```python
from build123d import *

# Parameters (mm, degrees)
F0_R        = 16.3870034363
F1_DEPTH    = 25.4
F2_T1_DEPTH = 116.4008158105
F2_T3_DEPTH = 104.7146316577
F2_T5_DEPTH = 112.6871608157
F2_T7_DEPTH = 79.0886539925
F3_T1_DEPTH = 116.4008158105
F3_T3_DEPTH = 104.7146316577
F3_T5_DEPTH = 112.6871608157
F3_T7_DEPTH = 79.0886539925


# Not quite as in the source:
# - a fillet or chamfer that OpenCascade refuses, or shapes differently, is made with other operations: its cross-section is extruded or revolved along the edge and cut away or added


with BuildPart() as f1:
    # F0 (on Top) → F1 (new body)
    with BuildSketch(Plane.XY):
        Polygon((27.1920096129, 8.1148929894), (-59.3668520451, 33.7408706546), (-59.3668520451, -44.8454618454), (27.1920096129, -44.8454618454), align=None)
        with Locations((0, -4.4133625925)):
            Circle(F0_R, mode=Mode.SUBTRACT)
    extrude(amount=F1_DEPTH)

    # F2: chamfer of 5.08 on 5 edges, made by hand

    # F2_s2 → F2_t1 (cut)
    with BuildSketch(Plane(origin=(35.3186398876, -10.4561758275, 0), x_dir=(0, 0, 1), z_dir=(-0.9588617319, 0.2838735267, 0))):
        Polygon((20.32, 15.5001520123), (25.4, 10.4201520123), (25.4, 15.5001520123), align=None)
    extrude(amount=F2_T1_DEPTH, mode=Mode.SUBTRACT)

    # F2_s4 → F2_t3 (cut)
    with BuildSketch(Plane.XZ.offset(-46.8050202334)):
        Polygon((-59.3668520451, 20.32), (-54.2868520451, 25.4), (-59.3668520451, 25.4), align=None)
    extrude(amount=F2_T3_DEPTH, mode=Mode.SUBTRACT)

    # F2_s6 → F2_t5 (cut)
    with BuildSketch(Plane.YZ.offset(-72.4310016239)):
        Polygon((-44.8454618454, 20.32), (-39.7654618454, 25.4), (-44.8454618454, 25.4), align=None)
    extrude(amount=F2_T5_DEPTH, mode=Mode.SUBTRACT)

    # F2_s8 → F2_t7 (cut)
    with BuildSketch(Plane.XZ.offset(-21.1790425683)):
        Polygon((27.1920096129, 20.32), (22.1120096129, 25.4), (27.1920096129, 25.4), align=None)
    extrude(amount=F2_T7_DEPTH, mode=Mode.SUBTRACT)

    # F2_s9 → F2_t10 (revolve, cut)
    with BuildSketch(Plane.XZ.offset(4.4133625925)):
        Polygon((16.3870034363, 20.32), (21.4670034363, 25.4), (16.3870034363, 25.4), align=None)
    revolve(axis=Axis((0, -4.4133625925, 25.4), (0, 0, 1)), mode=Mode.SUBTRACT)

    # F3: chamfer of 5.08 on 5 edges, made by hand

    # F3_s2 → F3_t1 (cut)
    with BuildSketch(Plane(origin=(35.3186398876, -10.4561758275, 0), x_dir=(0, 0, 1), z_dir=(-0.9588617319, 0.2838735267, 0))):
        Polygon((5.08, 15.5001520123), (0, 10.4201520123), (0, 15.5001520123), align=None)
    extrude(amount=F3_T1_DEPTH, mode=Mode.SUBTRACT)

    # F3_s4 → F3_t3 (cut)
    with BuildSketch(Plane.XZ.offset(-46.8050202334)):
        Polygon((-54.2868520451, 0), (-59.3668520451, 5.08), (-59.3668520451, 0), align=None)
    extrude(amount=F3_T3_DEPTH, mode=Mode.SUBTRACT)

    # F3_s6 → F3_t5 (cut)
    with BuildSketch(Plane.YZ.offset(-72.4310016239)):
        Polygon((-39.7654618454, 0), (-44.8454618454, 5.08), (-44.8454618454, 0), align=None)
    extrude(amount=F3_T5_DEPTH, mode=Mode.SUBTRACT)

    # F3_s8 → F3_t7 (cut)
    with BuildSketch(Plane.XZ.offset(-21.1790425683)):
        Polygon((22.1120096129, 0), (27.1920096129, 5.08), (27.1920096129, 0), align=None)
    extrude(amount=F3_T7_DEPTH, mode=Mode.SUBTRACT)

    # F3_s9 → F3_t10 (revolve, cut)
    with BuildSketch(Plane.XZ.offset(4.4133625925)):
        Polygon((21.4670034363, 0), (16.3870034363, 5.08), (16.3870034363, 0), align=None)
    revolve(axis=Axis((0, -4.4133625925, 0), (0, 0, 1)), mode=Mode.SUBTRACT)


solid = f1.part
```
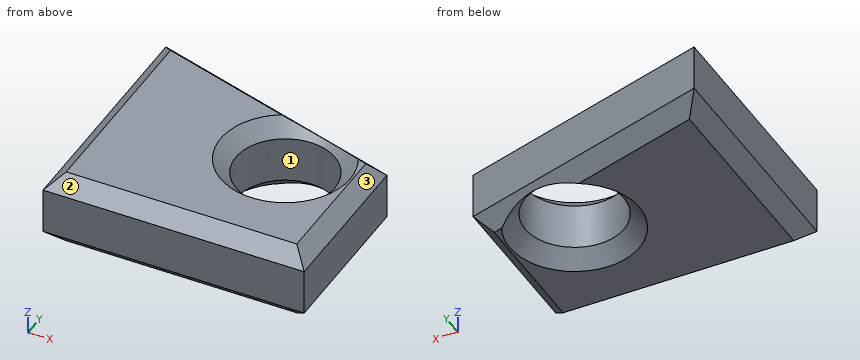
Part model, mm, in its own coordinate system. Face numbers are marked on the shaded views. Round coordinates to 2 decimals unless told otherwise and drop trailing zeros. Loops run counter-clockwise (first coordinate to the right, second up) from the corner with the lowest first, then second, coordinate; pieces in that order, holes last.
Item 1: Cut at C-C, the plane x = -49.5. Give the cut face in (y, z).
Item 2: Drop flat-ended pins along their axis: P1, Ø3, axis at x = 8, y = -18, coming from the +Z side; P2, Ø2, axis at x = -11.5, z = 10.5, coming from the +Y side; P3, Ø5, axis at x = -2.5, z = 7.5, coming from the +Y side. Give the stop position or say it passes through.
Item 3: Cut at B-B, the plane y = -33. Give the cut face in (x, z), then the cut area to 3 significant figures.
Item 4: Drill centre lines: line 1 (Y direction, x = 0, z = 8.75); line 2 (X direction, y = -3, z = 8.25); line 3 (X direction, y = 8, z = 16.5). Where is each one in solid material? Low to high.
Item 5: Cut at D-D, the plane z = 8.5. Give the cut face in (x, y), then the cut area to 3 significant figures.
Item 6: Mould opens along Y. For the marked faces 1, 2 and 3 say: +Y half, -Y half, draft (parallel to the pull), parting line (faces both ways), or undercut.
Item 7: Cut at A-A, the plane x = 0. Give the cut face in (y, z), then the cut area to 3 significant figures.
A:
1. outline: (-44.85, 5.08) - (-39.77, 0) - (25.52, 0) - (30.82, 5.08) - (30.82, 20.32) - (25.52, 25.4) - (-39.77, 25.4) - (-44.85, 20.32) - close
2. P1: stops at z = 21.2
2. P2: stops at y = 19.87
2. P3: stops at y = 17.65
3. outline: (-59.37, 5.08) - (-54.29, 0) - (22.11, 0) - (27.19, 5.08) - (27.19, 20.32) - (22.11, 25.4) - (-54.29, 25.4) - (-59.37, 20.32) - close
3. area: 2,150 mm2
4. line 1: y = -44.85 to -20.8, 11.97 to 16.17
4. line 2: x = -59.37 to -16.33, 16.33 to 27.19
4. line 3: x = -59.37 to -10.7, 10.7 to 27.19
5. outline: (-59.37, -44.85) - (27.19, -44.85) - (27.19, 8.11) - (-59.37, 33.74) - close; hole circle Ø32.77 at (0, -4.41)
5. area: 4,850 mm2
6. face 1: undercut
6. face 2: -Y half
6. face 3: draft
7. outline: (-44.85, 5.08) - (-39.77, 0) - (-25.88, 0) - (-20.8, 5.08) - (-20.8, 20.32) - (-25.88, 25.4) - (-39.77, 25.4) - (-44.85, 20.32) - close; (11.97, 5.08) - (14.03, 3.03) - (16.17, 5.08) - (16.17, 20.32) - (14.03, 22.37) - (11.97, 20.32) - close
7. area: 632 mm2
